```python
from build123d import *

# Parameters (mm, degrees)
F1_DEPTH      = 20
F2_W          = 7.5
F2_H          = 1
F3_DEPTH      = 2.5
F5_DEPTH      = 1
F7_DEPTH      = 20
F10_DEPTH     = 19
F12_DEPTH     = 0.5
F14_DEPTH     = 0.5
F15_R         = 7
F15_R_2       = 3.2
F16_DEPTH     = 2
F17_SIZE      = 1.99999
F18_R         = 1.5
F19_DEPTH     = 2
F20_R         = 2.5
F21_DEPTH     = 2
F22_W         = 6
F22_H         = 4
F23_DEPTH     = 6
F24_T1_DEPTH  = 34.6
F24_T3_DEPTH  = 7.5
F24_T5_DEPTH  = 38.5
F24_T7_DEPTH  = 18
F24_T9_DEPTH  = 6
F24_T11_DEPTH = 6
F24_S15_W     = 1
F24_S15_H     = 1
F24_T16_DEPTH = 1
F24_S21_W     = 1
F24_S21_H     = 1
F24_T22_DEPTH = 1
F24_S27_W     = 1
F24_S27_H     = 1
F24_T28_DEPTH = 1
F24_S33_W     = 1
F24_S33_H     = 1
F24_T34_DEPTH = 1


# Not quite as in the source:
# - a fillet or chamfer that OpenCascade refuses, or shapes differently, is made with other operations: its cross-section is extruded or revolved along the edge and cut away or added
# - a fillet or chamfer is up to 0.001 mm smaller than in the source, because OpenCascade refuses the exact size


with BuildPart() as f1:
    # F0 (on Front) → F1 (new body)
    with BuildSketch(Plane.XZ):
        Polygon((0, 26.6), (0, 0), (40.5, 0), (40.5, 26.6), (48, 26.6), (48, 29.1), (40.5, 29.1), (40.5, 36.1), (0, 36.1), (0, 29.1), (-7.5, 29.1), (-7.5, 26.6), align=None)
    extrude(amount=F1_DEPTH)

    # F2 (on face) → F3 (cut, through all)
    with BuildSketch(Plane.XY.offset(29.1)):
        with Locations((-3.75, -0.5)):
            Rectangle(F2_W, F2_H)
        with Locations((-3.75, -19.5)):
            Rectangle(F2_W, F2_H)
        with BuildLine():
            ThreePointArc((-7.5, -6.6), (-7.2314497593, -6.2261647771), (-6.7914469101, -6.3613294855))
            ThreePointArc((-6.7914469101, -6.3613294855), (-2.75, -5), (-6.7914469101, -3.6386705145))
            ThreePointArc((-6.7914469101, -3.6386705145), (-7.2314497593, -3.7738352229), (-7.5, -3.4))
            Line((-7.5, -3.4), (-7.5, -6.6))
        make_face()
        with BuildLine():
            ThreePointArc((-7.5, -16.6), (-7.2314497593, -16.2261647771), (-6.7914469101, -16.3613294855))
            ThreePointArc((-6.7914469101, -16.3613294855), (-2.75, -15), (-6.7914469101, -13.6386705145))
            ThreePointArc((-6.7914469101, -13.6386705145), (-7.2314497593, -13.7738352229), (-7.5, -13.4))
            Line((-7.5, -13.4), (-7.5, -16.6))
        make_face()
        with BuildLine():
            Line((48, -16.6), (48, -13.4))
            ThreePointArc((48, -13.4), (47.7314497593, -13.7738352229), (47.2914469101, -13.6386705145))
            ThreePointArc((47.2914469101, -13.6386705145), (43.25, -15), (47.2914469101, -16.3613294855))
            ThreePointArc((47.2914469101, -16.3613294855), (47.7314497593, -16.2261647771), (48, -16.6))
        make_face()
        with Locations((44.25, -0.5)):
            Rectangle(F2_W, F2_H)
        with BuildLine():
            ThreePointArc((47.2914469101, -3.6386705145), (43.25, -5), (47.2914469101, -6.3613294855))
            ThreePointArc((47.2914469101, -6.3613294855), (47.7314497593, -6.2261647771), (48, -6.6))
            Line((48, -6.6), (48, -3.4))
            ThreePointArc((48, -3.4), (47.7314497593, -3.7738352229), (47.2914469101, -3.6386705145))
        make_face()
        with Locations((44.25, -19.5)):
            Rectangle(F2_W, F2_H)
    extrude(amount=-F3_DEPTH, mode=Mode.SUBTRACT)

    # F4 (on face) → F5 (join)
    with BuildSketch(Plane.XY.offset(29.1)):
        with BuildLine():
            Line((0, -11), (0, -9))
            Line((0, -9), (-3, -9))
            ThreePointArc((-3, -9), (-4, -10), (-3, -11))
            Line((-3, -11), (0, -11))
        make_face()
        with BuildLine():
            Line((43.5, -9), (40.5, -9))
            Line((40.5, -9), (40.5, -11))
            Line((40.5, -11), (43.5, -11))
            ThreePointArc((43.5, -11), (44.5, -10), (43.5, -9))
        make_face()
    extrude(amount=F5_DEPTH)

    # F6 (on face) → F7 (cut, through all)
    with BuildSketch(Plane.XZ.offset(20)):
        Polygon((40.5, 36.1), (0, 36.1), (0, 33.1), (18.1, 35.6), (38, 35.6), (40.5, 33.1), align=None)
    extrude(amount=-F7_DEPTH, mode=Mode.SUBTRACT)

    # F9 (on offset) → F10 (join)
    with BuildSketch(Plane.XZ.offset(19.5)):
        Polygon((5.5856353591, 36.1), (3, 33.5143646409), (18.1, 35.6), (18.7, 35.6), (18.7, 36.1), align=None)
        Polygon((39.5, 36.1), (19.7, 36.1), (19.7, 35.6), (38, 35.6), (40.5, 33.1), align=None)
    extrude(amount=-F10_DEPTH)

    # F11 (on face) → F12 (cut, through all)
    with BuildSketch(Plane.XY.offset(36.1)):
        with BuildLine():
            Line((19.7, -7), (19.7, -13))
            ThreePointArc((19.7, -13), (21.8622776602, -10), (19.7, -7))
        make_face()
    extrude(amount=-F12_DEPTH, mode=Mode.SUBTRACT)

    # F13 (on face) → F14 (join)
    with BuildSketch(Plane.XY.offset(35.6)):
        with BuildLine():
            Line((18.7, -7.8377223398), (18.7, -12.1622776602))
            ThreePointArc((18.7, -12.1622776602), (20.8622776602, -10), (18.7, -7.8377223398))
        make_face()
    extrude(amount=F14_DEPTH)

    # F15 (on face) → F16 (join)
    with BuildSketch(Plane.XY.offset(36.1)):
        with Locations((30.1, -10)):
            Circle(F15_R)
        with Locations((30.1, -10)):
            Circle(F15_R_2, mode=Mode.SUBTRACT)
    extrude(amount=F16_DEPTH)

    # F17 (size 2 in the source; OpenCascade refuses exactly that, so slightly less here)
    f17_edges = [f1.edges().sort_by_distance(p)[0] for p in [
        (23.1, -10, 38.1),
    ]]
    chamfer(f17_edges, length=F17_SIZE)

    # F18 (on face) → F19 (cut)
    with BuildSketch(Plane.XY.offset(36.1)):
        with Locations((30.1, -10)):
            Circle(F18_R)
    extrude(amount=-F19_DEPTH, mode=Mode.SUBTRACT)

    # F20 (on face) → F21 (cut)
    with BuildSketch(Plane.YZ.offset(40.5)):
        with Locations((-10, 9.5)):
            Circle(F20_R)
    extrude(amount=-F21_DEPTH, mode=Mode.SUBTRACT)

    # F22 (on face) → F23 (join)
    with BuildSketch(Plane.YZ.offset(40.5)):
        with Locations((-10, 2)):
            Rectangle(F22_W, F22_H)
    extrude(amount=F23_DEPTH)

    # F24: fillet of radius 1 on 13 edges, made by hand

    # F24_s2 → F24_t1 (cut)
    with BuildSketch(Plane.XY.offset(1)):
        with BuildLine():
            ThreePointArc((1, 0), (0.2928932188, -0.2928932188), (0, -1))
            Line((0, -1), (0, 0))
            Line((0, 0), (1, 0))
        make_face()
        with BuildLine():
            ThreePointArc((1, -20), (0.2928932188, -19.7071067812), (0, -19))
            Line((0, -19), (0, -20))
            Line((0, -20), (1, -20))
        make_face()
        with BuildLine():
            ThreePointArc((40.5, -19), (40.2071067812, -19.7071067812), (39.5, -20))
            Line((39.5, -20), (40.5, -20))
            Line((40.5, -20), (40.5, -19))
        make_face()
        with BuildLine():
            ThreePointArc((40.5, -1), (40.2071067812, -0.2928932188), (39.5, 0))
            Line((39.5, 0), (40.5, 0))
            Line((40.5, 0), (40.5, -1))
        make_face()
    extrude(amount=F24_T1_DEPTH, mode=Mode.SUBTRACT)

    # F24_s4 → F24_t3 (cut)
    with BuildSketch(Plane.XY.offset(24.1)):
        with BuildLine():
            ThreePointArc((-6.5, -19), (-7.2071067812, -18.7071067812), (-7.5, -18))
            Line((-7.5, -18), (-7.5, -19))
            Line((-7.5, -19), (-6.5, -19))
        make_face()
        with BuildLine():
            ThreePointArc((-6.5, -1), (-7.2071067812, -1.2928932188), (-7.5, -2))
            Line((-7.5, -2), (-7.5, -1))
            Line((-7.5, -1), (-6.5, -1))
        make_face()
        with BuildLine():
            ThreePointArc((47, -1), (47.7071067812, -1.2928932188), (48, -2))
            Line((48, -2), (48, -1))
            Line((48, -1), (47, -1))
        make_face()
        with BuildLine():
            ThreePointArc((47, -19), (47.7071067812, -18.7071067812), (48, -18))
            Line((48, -18), (48, -19))
            Line((48, -19), (47, -19))
        make_face()
    extrude(amount=F24_T3_DEPTH, mode=Mode.SUBTRACT)

    # F24_s6 → F24_t5 (cut)
    with BuildSketch(Plane.YZ.offset(1)):
        with BuildLine():
            ThreePointArc((-20, 1), (-19.7071067812, 0.2928932188), (-19, 0))
            Line((-19, 0), (-20, 0))
            Line((-20, 0), (-20, 1))
        make_face()
        with BuildLine():
            ThreePointArc((0, 1), (-0.2928932188, 0.2928932188), (-1, 0))
            Line((-1, 0), (0, 0))
            Line((0, 0), (0, 1))
        make_face()
    extrude(amount=F24_T5_DEPTH, mode=Mode.SUBTRACT)

    # F24_s8 → F24_t7 (cut)
    with BuildSketch(Plane.XZ.offset(1)):
        with BuildLine():
            ThreePointArc((1, 0), (0.2928932188, 0.2928932188), (0, 1))
            Line((0, 1), (0, 0))
            Line((0, 0), (1, 0))
        make_face()
    extrude(amount=F24_T7_DEPTH, mode=Mode.SUBTRACT)

    # F24_s10 → F24_t9 (cut)
    with BuildSketch(Plane.XZ.offset(13)):
        with BuildLine():
            ThreePointArc((40.5, 1), (40.2071067812, 0.2928932188), (39.5, 0))
            Line((39.5, 0), (40.5, 0))
            Line((40.5, 0), (40.5, 1))
        make_face()
    extrude(amount=F24_T9_DEPTH, mode=Mode.SUBTRACT)

    # F24_s12 → F24_t11 (cut)
    with BuildSketch(Plane.XZ.offset(1)):
        with BuildLine():
            ThreePointArc((40.5, 1), (40.2071067812, 0.2928932188), (39.5, 0))
            Line((39.5, 0), (40.5, 0))
            Line((40.5, 0), (40.5, 1))
        make_face()
    extrude(amount=F24_T11_DEPTH, mode=Mode.SUBTRACT)


with BuildPart() as f24_tool14:
    # F24_s15 → F24_t16 (new body)
    with BuildSketch(Plane.XY.offset(1)):
        with Locations((0.5, -0.5)):
            Rectangle(F24_S15_W, F24_S15_H)
    extrude(amount=-F24_T16_DEPTH)

    # F24_s17 → F24_t18 (revolve, cut)
    with BuildSketch(Plane(origin=(1, -1, 1), x_dir=(0.7071067812, -0.7071067812, 0), z_dir=(0.7071067812, 0.7071067812, 0))):
        with BuildLine():
            ThreePointArc((0, -1), (1, 0), (0, 1))
            Line((0, 1), (0, -1))
        make_face()
    revolve(axis=Axis((1, -1, 1), (0, 0, -1)), mode=Mode.SUBTRACT)


with BuildPart() as f1_1:
    add(f1.part)

    # F24_t13: cut F24_tool14
    add(f24_tool14.part, mode=Mode.SUBTRACT)


with BuildPart() as f24_tool20:
    # F24_s21 → F24_t22 (new body)
    with BuildSketch(Plane.XZ.offset(19)):
        with Locations((0.5, 0.5)):
            Rectangle(F24_S21_W, F24_S21_H)
    extrude(amount=F24_T22_DEPTH)

    # F24_s23 → F24_t24 (revolve, cut)
    with BuildSketch(Plane(origin=(1, -19, 1), x_dir=(0.7071067812, 0, 0.7071067812), z_dir=(0.7071067812, 0, -0.7071067812))):
        with BuildLine():
            ThreePointArc((0, -1), (1, 0), (0, 1))
            Line((0, 1), (0, -1))
        make_face()
    revolve(axis=Axis((1, -19, 1), (0, -1, 0)), mode=Mode.SUBTRACT)


with BuildPart() as f1_2:
    add(f1_1.part)

    # F24_t19: cut F24_tool20
    add(f24_tool20.part, mode=Mode.SUBTRACT)


with BuildPart() as f24_tool26:
    # F24_s27 → F24_t28 (new body)
    with BuildSketch(Plane.XZ.offset(19)):
        with Locations((40, 0.5)):
            Rectangle(F24_S27_W, F24_S27_H)
    extrude(amount=F24_T28_DEPTH)

    # F24_s29 → F24_t30 (revolve, cut)
    with BuildSketch(Plane(origin=(39.5, -19, 1), x_dir=(-0.7071067812, 0, 0.7071067812), z_dir=(0.7071067812, 0, 0.7071067812))):
        with BuildLine():
            ThreePointArc((0, -1), (1, 0), (0, 1))
            Line((0, 1), (0, -1))
        make_face()
    revolve(axis=Axis((39.5, -19, 1), (0, -1, 0)), mode=Mode.SUBTRACT)


with BuildPart() as f1_3:
    add(f1_2.part)

    # F24_t25: cut F24_tool26
    add(f24_tool26.part, mode=Mode.SUBTRACT)


with BuildPart() as f24_tool32:
    # F24_s33 → F24_t34 (new body)
    with BuildSketch(Plane.XY.offset(1)):
        with Locations((40, -0.5)):
            Rectangle(F24_S33_W, F24_S33_H)
    extrude(amount=-F24_T34_DEPTH)

    # F24_s35 → F24_t36 (revolve, cut)
    with BuildSketch(Plane(origin=(39.5, -1, 1), x_dir=(-0.7071067812, -0.7071067812, 0), z_dir=(0.7071067812, -0.7071067812, 0))):
        with BuildLine():
            ThreePointArc((0, -1), (1, 0), (0, 1))
            Line((0, 1), (0, -1))
        make_face()
    revolve(axis=Axis((39.5, -1, 1), (0, 0, -1)), mode=Mode.SUBTRACT)


with BuildPart() as f1_4:
    add(f1_3.part)

    # F24_t31: cut F24_tool32
    add(f24_tool32.part, mode=Mode.SUBTRACT)


solid = f1_4.part
```
Can you work these out from the model? Positions are in its coordinate system, mm. A direction names the side the tool comes from. Give positions to 0.01 mm unless a question says otherwise; leave off trailing zeros. Loops run counter-clockwise (first coordinate to the right, second up) from the corner with the lowest first, then second, coordinate; pieces in that order, holes last. Notation, with made-up numbers: M -9,68 L 4,68 A18 cw 4,94 Z; hole C 54.5,-38.5 d8. An arc over 180 degrees is marked long. Use one line per item in the form item = value. Start each with the question number.
(1) On a 3-axis mill with a long thin cutter (end or side, diameter ignored), from which of +Z, -Z, +X, -X, +Y, -Y can I reach the whole of each face in a straight line? I mean faces 1 (the flat face through (38.5, -10, 10)), 2 (the flat face through (45, -10, 29.1)), 3 (the cylindrical face through (28.6, -9.93, 35.11)). Say none if no direction works.
(2) I'm going to push flat-ended pins straight in: P1, Ø0.8, axis at x = 43, z = 27.5, coming from the -Y side; P2, Ø4.5, axis at x = 10.5, y = -12.5, coming from the +Z side; P3, Ø4, axis at y = -7, z = 10, coming from the +X side; P4, Ø10, axis at x = 30.1, y = -10, coming from the +Z side. Where does each tip first touch, or does it pass through?
(3) I want a section at D-D, the plane x = 14. Write out the boundary of the cut face in (y, z).
(4) I want a section at C-C, the plane x = -1. Write out the boundary of the cut face in (y, z).
(5) Thinking about a two-plate mould opening in Y: for faces 4 (the cylindrical face through (20.86, -10.05, 35.85)), 5 (the flat face through (44, -7, 2)), 6 (the flat face through (31.5, -19.5, 35.9)), 7 (the flat face through (-3, -10, 26.6)), which applies, released by +Y, released by -Y, zero draft, split by the parting line, or undercut?
(6) I want a section at B-B, the plane z = 9.5. Write out the boundary of the cut face in (x, y), and give its area (3 significant figures).
(7) Please list where these lines run through material, in increasing order: line 1 (Y direction, x = 45.5, z = 27.35); line 2 (Y direction, x = 30.1, z = 35.05); line 3 (Z direction, x = 34, y = -18.75).
Worked out:
q1.face_1 = +X
q1.face_2 = +Z, +X
q1.face_3 = +Z
q2.P1 = -19
q2.P2 = 36.1
q2.P3 = 40.5
q2.P4 = 38.1
q3.outline = M -20,1 A1 ccw -19,0 L -1,0 A1 ccw 0,1 L 0,35.03 L -0.5,35.03 L -0.5,36.1 L -19.5,36.1 L -19.5,35.03 L -20,35.03 Z
q4.outline = M -19,26.6 L -1,26.6 L -1,29.1 L -9,29.1 L -9,30.1 L -11,30.1 L -11,29.1 L -19,29.1 Z
q5.face_4 = undercut
q5.face_5 = released by +Y
q5.face_6 = released by -Y
q5.face_7 = zero draft
q6.outline = M 0,-19 A1 ccw 1,-20 L 39.5,-20 A1 ccw 40.5,-19 L 40.5,-12.5 L 38.5,-12.5 L 38.5,-7.5 L 40.5,-7.5 L 40.5,-1 A1 ccw 39.5,0 L 1,0 A1 ccw 0,-1 Z
q6.area = 799 mm²
q7.line_1 = -19 to -17.25, -12.75 to -7.25, -2.75 to -1
q7.line_2 = -20 to -11.5, -8.5 to 0
q7.line_3 = 0 to 36.1
